Solid Edge part; units mm, degrees
sketch "Sketch1" plane through (0, 0, 0) normal (0, -1, 0) x (1, 0, 0)
  line L0 (300, 40) -> (130, 40)
  line L1 (130, 40) -> (0, 5)
  line L2 (0, 0) -> (0, 5)
  line L3 (0, 0) -> (300, 0)
  line L4 (300, 0) -> (300, 10)
  line L5 (300, 10) -> (130, 10)
  line L6 (130, 10) -> (130, 30)
  line L7 (130, 30) -> (300, 30)
  line L8 (300, 30) -> (300, 40)
extrude "Protrusion1" add sketch "Sketch1" against normal blind 60
sketch "Sketch2" plane through (459.6291, 50, 40) normal (0, 0, 1) x (1, 0, 0)
  circle A0 centre (-259.6291, -20) radius 15
  circle A1 centre (-184.6291, -20) radius 15
extrude "Cutout1" cut sketch "Sketch2" against normal through all
sketch "Sketch3" plane through (459.6291, 50, 40) normal (0, 0, 1) x (0, 1, 0)
  line L0 (-40, 339.6291) -> (0, 339.6291)
  line L1 (0, 339.6291) -> (0, 459.6291)
  line L2 (0, 459.6291) -> (-40, 459.6291)
  line L3 (-40, 459.6291) -> (-40, 339.6291)
  dimension "D1" = 40
extrude "ExtrudedCutout_2" cut sketch "Sketch3" against normal blind 35
fillet "Round_1" radius 5 4 edges at (300, 0, 5) (300, 60, 5) (300, 60, 35) (300, 0, 35)
fillet "Round_2" radius 20 1 edges at (130, 30, 40)
sketch "Sketch4" plane through (150, 40, 0) normal (0, 0, -1) x (1, 0, 0)
  line L0 (150, -15) -> (50, -15)
  line L1 (150, 35) -> (50, 35)
  line L2 (150, 35) -> (150, -15)
  arc A0 (50, -15) -> (50, 35) centre (50, 10) cw
  dimension "D1" = 150
  dimension "D2" = 150
extrude "ExtrudedCutout_3" cut sketch "Sketch4" against normal blind 5
Check sheet for the modelled part. Datum: model origin and axes. Units: mm. A direction names the side the tool comes from. Give positions to 0.01 mm unless a question says otherwise; leave off trailing zeros. Loops run counter-clockwise (first coordinate to the right, second up) from the corner with the lowest first, then second, coordinate; pieces in that order, holes last. Notation, with made-up numbers: M 47,-34.5 L 76,-34.5 A24 ccw 76,-5.5 Z; hole C -19,24.5 d10. An arc over 180 degrees is marked long. Answer in a Markdown table with one row per item.
1) Mould release check, pull along Y, two halves, no side actions. Record for faces 6 (the face through (130, 30, 20)), 7 (the face through (74, 50, 18)), 8 (the face through (237, 30, 5)), 9 (the face through (298, 1, 35)): released by +Y, released by -Y, zero draft, split by the parting line, or undercut.
Solutions:
| item | result |
|---|---|
| face 6 | zero draft |
| face 7 | undercut |
| face 8 | undercut |
| face 9 | released by -Y |
2) Cross-section at A-A (y = 30). Count the separate pieces of the cut face and the enclosed holes in it, plus the area to 3 significant figures.
Solutions:
| item | result |
|---|---|
| separate pieces | 5 |
| enclosed holes | 0 |
| area | 2,860 mm^2 |
3) Cross-section at D-D (x = 26). Enter the section's corners in (y, z), plus the area to 3 significant figures.
Solutions:
| item | result |
|---|---|
| outline | M 0,0 L 60,0 L 60,12 L 50,12 L 50,5 L 10,5 L 10,12 L 0,12 Z |
| area | 440 mm^2 |
4) Tool access check on faces 1 (the face through (251, 5, 2)), 2 (the face through (78.78, 9.58, 26.21)), 3 (the face through (214, 36, 30)), 4 (the face through (86, 10, 14)), 5 (the face through (299, 58, 35)). Record the directions out of +Z, -Z, +X, -X, +Y, -Y that give a thin tool (end or side, any length) a straight path to the whole face; none if there is none.
Solutions:
| item | result |
|---|---|
| face 1 | -Z, +X |
| face 2 | +Z, -X, +Y, -Y |
| face 3 | +X, +Y, -Y |
| face 4 | +Z, -X |
| face 5 | +Z, -Z, +X, +Y |
5) Depth check by flat-ended pin: pin 1 (5 mm diameter, centred on y = 26.5, z = 14, fed in from +X); pin 2 (6 mm diameter, centred on y = 17.5, z = 31, fed in from -X); pin 3 (4 mm diameter, centred on x = 82, y = 53.5, fed in from +Z); pin 4 (18 mm diameter, centred on x = 200, y = 30, fed in from -Z). Enter the tip coordinate at first touch or a pass-through.
Solutions:
| item | result |
|---|---|
| pin 1 | stops at x = 130 |
| pin 2 | stops at x = 120 |
| pin 3 | stops at z = 27.62 |
| pin 4 | passes through |
6) Cross-section at B-B (x = 275). Enter the section's corners in (y, z), plus the area to 3 significant figures.
Solutions:
| item | result |
|---|---|
| outline | M 0,0 L 5,0 L 5,5 L 15,5 L 15,10 L 0,10 Z; M 0,30 L 15,30 L 15,40 L 0,40 Z; M 45,5 L 55,5 L 55,0 L 60,0 L 60,10 L 45,10 Z; M 45,30 L 60,30 L 60,40 L 45,40 Z |
| area | 500 mm^2 |
7) Thickness scan on line 1 (Z direction, x = 272, y = 47); line 2 (Y direction, x = 200, z = 6); line 3 (Z direction, x = 135.5, y = 42). Record the ranges inside material, lowest first.
Solutions:
| item | result |
|---|---|
| line 1 | z = 5 to 10, 30 to 40 |
| line 2 | y = 0 to 15, 45 to 60 |
| line 3 | z = 0 to 10, 30 to 40 |
8) Cross-section at C-C (x = 151). Enter the section's corners in (y, z), plus the area to 3 significant figures.
Solutions:
| item | result |
|---|---|
| outline | M 0,0 L 60,0 L 60,10 L 0,10 Z; M 0,30 L 60,30 L 60,40 L 0,40 Z |
| area | 1,200 mm^2 |
